Could you check a few things on this model? Use its own coordinates, in mm. Face numbers are marked on the shaded views. Give positions to 0.01 mm unless a question says otherwise; leave off trailing zeros. Order: outer loops, then holes, each group sorted by start corner. A loop starts at its lowest first (then second) coordinate and runs counter-clockwise, first axis right, second up. Notation, with made-up numbers: (41, -4) -> (48, -4) arc R15 cw to (48, 8) -> close; hole circle Ø6 at (73, -32). An arc over 180 degrees is marked (long way). Write each question's results on one line, items separated by ' | '.
```python
from build123d import *

# Parameters (mm, degrees)
BOSS_EXTRUDE1_DEPTH                          = 60
FILLET1_R                                    = 3
CBORE_FOR_M5_HEX_SOCKET_HEAD_CAP_SCR_2_COUNT = 2
CBORE_FOR_M5_HEX_SOCKET_HEAD_CAP_SCR_2_PITCH = 19


with BuildPart() as part:
    # Sketch1 → Boss-Extrude1 (new body)
    with BuildSketch(Plane.XY):
        Polygon((-20.5, 0), (-13.57179677, 12), (13.57179677, 12), (20.5, 0), align=None)
    extrude(amount=BOSS_EXTRUDE1_DEPTH)

    # Fillet1
    fillet1_edges = [part.edges().sort_by_distance(p)[0] for p in [
        (0, 12, 60),
        (-17.035898385, 6, 60),
        (0, 0, 60),
        (-17.035898385, 6, 0),
        (0, 12, 0),
        (17.035898385, 6, 0),
        (0, 0, 0),
        (-13.57179677, 12, 30),
        (13.57179677, 12, 30),
        (17.035898385, 6, 60),
    ]]
    fillet(fillet1_edges, radius=FILLET1_R)

    # Sketch5 → CBORE for M5 Hex Socket Head Cap Screw1 (revolve, cut)
    with BuildSketch(Plane(origin=(9.5, 0, 30), x_dir=(0, 0, -1), z_dir=(1, 0, 0))):
        Polygon((0, 0), (0, 12), (2.75, 12), (2.75, 5.4), (5, 5.4), (5, 0.025), (5.025, 0), align=None)
    cbore_for_m5_hex_socket_head_cap_screw1 = revolve(axis=Axis((9.5, -6.35, 30), (0, 1, 0)), mode=Mode.SUBTRACT)

    # CBORE for M5 Hex Socket Head Cap Scr 2: CBORE for M5 Hex Socket Head Cap Screw1 ×2
    with Locations(*[(-i * CBORE_FOR_M5_HEX_SOCKET_HEAD_CAP_SCR_2_PITCH, 0, 0) for i in range(1, CBORE_FOR_M5_HEX_SOCKET_HEAD_CAP_SCR_2_COUNT)]):
        add(cbore_for_m5_hex_socket_head_cap_screw1, mode=Mode.SUBTRACT)


solid = part.part
```
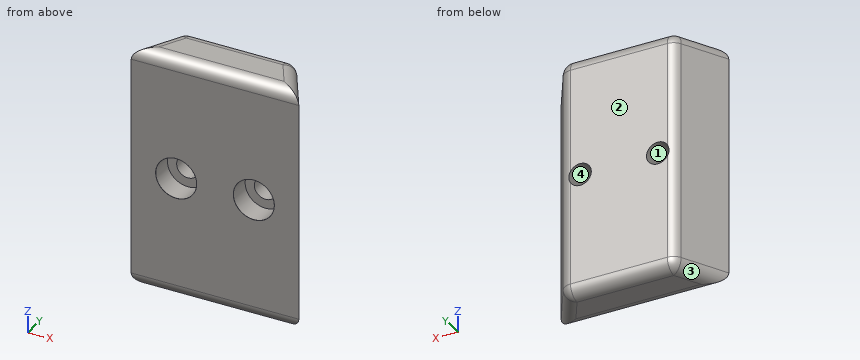
Q1. I need wall thicknesses on line 1 along Z through (x, y) = (-9.5, 3.9); line 2 along X through (y, z) = (2.2, 30); line 3 along X through (y, z) = (10, 30). Which ranges of each line are inside material? Lowest first, please.
Here are the results:
line 1: z = 0 to 25, 35 to 60 | line 2: x = -19.23 to -14.5, -4.5 to 4.5, 14.5 to 19.23 | line 3: x = -14.73 to -12.25, -6.75 to 6.75, 12.25 to 14.73
Q2. I'm going to push flat-ended pins straight in: pin 1 Ø9 at (x, z) = (-9.5, 30) entering from -Y; pin 2 Ø3 at (x, z) = (9, 31) entering from -Y; pin 3 Ø3 at (y, z) = (6.5, 42.5) entering from +X; pin 4 Ø4 at (y, z) = (7, 14) entering from -X. Where does each tip first touch, or does it pass through?
Here are the results:
pin 1: stops at y = 5.4 | pin 2: passes through | pin 3: stops at x = 17.61 | pin 4: stops at x = -17.61
Q3. Suppose I cut it at D-D on y = 2.25. State how many separate pieces and enclosed holes the cut face has, and give its area (3 significant figures).
Here are the results:
separate pieces: 1 | enclosed holes: 2 | area: 2,130 mm²
Q4. Suppose I cut it at B-B on z = 30. Please give me the cut outline in (x, y) (3 decimals).
Here are the results:
outline: (-20.5, 0) -> (-14.525, 0) -> (-14.5, 0.025) -> (-14.5, 5.4) -> (-12.25, 5.4) -> (-12.25, 11.972) arc R3 ccw to (-14.438, 10.5) -> close; (-6.75, 5.4) -> (-4.5, 5.4) -> (-4.5, 0.025) -> (-4.475, 0) -> (4.475, 0) -> (4.5, 0.025) -> (4.5, 5.4) -> (6.75, 5.4) -> (6.75, 12) -> (-6.75, 12) -> close; (12.25, 5.4) -> (14.5, 5.4) -> (14.5, 0.025) -> (14.525, 0) -> (20.5, 0) -> (14.438, 10.5) arc R3 ccw to (12.25, 11.972) -> close
Q5. Suppose I cut it at A-A on x = -9.5. Please give me the cut outline in (y, z) (3 decimals), and give its area (3 significant figures).
Here are the results:
outline: (0, 3) arc R3 ccw to (3, 0) -> (9, 0) arc R3 ccw to (12, 3) -> (12, 27.25) -> (5.4, 27.25) -> (5.4, 25) -> (0.025, 25) -> (0, 24.975) -> close; (0, 35.025) -> (0.025, 35) -> (5.4, 35) -> (5.4, 32.75) -> (12, 32.75) -> (12, 57) arc R3 ccw to (9, 60) -> (3, 60) arc R3 ccw to (0, 57) -> close | area: 622 mm²
Q6. Thinking about a two-plate mould opening in Z: for the marked faces 1, 2, 3 and 4, which applies, +Z half, -Z half, draft (parallel to the pull), parting line (faces both ways), or undercut?
Here are the results:
face 1: undercut | face 2: draft | face 3: -Z half | face 4: undercut
Q7. Suppose I cut it at C-C on z = 19.5. Please give me the cut outline in (x, y).
Here are the results:
outline: (-20.5, 0) -> (20.5, 0) -> (14.44, 10.5) arc R3 ccw to (11.84, 12) -> (-11.84, 12) arc R3 ccw to (-14.44, 10.5) -> close
